from build123d import *

# Parameters (mm, degrees)
F0_R        = 1.1
F1_DEPTH    = 4.75
F2_R        = 5
F3_DEPTH    = 5
F5_T1_DEPTH = 16.1499020619
F5_T3_DEPTH = 14.3297238483
F5_T5_DEPTH = 10.7226436636
F7_DEPTH    = 0.8
F8_R        = 0.75
F9_R        = 9.625
F10_DEPTH   = 3
F12_R       = 4.5172071506
F12_R_2     = 2.2672071506
F13_DEPTH   = 3.7


# Not quite as in the source:
# - a fillet or chamfer that OpenCascade refuses, or shapes differently, is made with other operations: its cross-section is extruded or revolved along the edge and cut away or added


with BuildPart() as f1:
    # F0 (on Top) → F1 (new body)
    with BuildSketch(Plane.XY):
        with BuildLine():
            Line((-8.3357166343, -1.6650899635), (-12.2050748298, -2.6992866465))
            ThreePointArc((-12.2050748298, -2.6992866465), (-9.3300068577, -8.3187121621), (-4.0757746589, -11.8168549509))
            ThreePointArc((-4.0757746589, -11.8168549509), (-3.593311946, -12.8676823003), (-2.8459674038, -13.75))
            Line((-2.8459674038, -13.75), (2.8459674038, -13.75))
            ThreePointArc((2.8459674038, -13.75), (3.593311946, -12.8676823003), (4.0757746589, -11.8168549509))
            ThreePointArc((4.0757746589, -11.8168549509), (9.3300068577, -8.3187121621), (12.2050748298, -2.6992866465))
            Line((12.2050748298, -2.6992866465), (8.3357166343, -1.6650899635))
            ThreePointArc((8.3357166343, -1.6650899635), (8.1313688943, -2.4774051544), (7.8480653995, -3.2656646917))
            ThreePointArc((7.8480653995, -3.2656646917), (8.5179809488, -4.8326547168), (6.82922604, -5.061459087))
            Line((6.82922604, -5.061459087), (5.0334316447, -3.2656646917))
            ThreePointArc((5.0334316447, -3.2656646917), (0, 6), (-5.0334316447, -3.2656646917))
            Line((-5.0334316447, -3.2656646917), (-6.82922604, -5.061459087))
            ThreePointArc((-6.82922604, -5.061459087), (-8.5179809488, -4.8326547168), (-7.8480653995, -3.2656646917))
            ThreePointArc((-7.8480653995, -3.2656646917), (-8.1313688943, -2.4774051544), (-8.3357166343, -1.6650899635))
        make_face()
        with Locations((0, -10.9)):
            Circle(F0_R, mode=Mode.SUBTRACT)
        with BuildLine():
            Line((-5.061459087, -6.82922604), (-3.2656646917, -5.0334316447))
            ThreePointArc((-3.2656646917, -5.0334316447), (0, -6), (3.2656646917, -5.0334316447))
            Line((3.2656646917, -5.0334316447), (5.061459087, -6.82922604))
            ThreePointArc((5.061459087, -6.82922604), (4.8326547168, -8.5179809488), (3.2656646917, -7.8480653995))
            ThreePointArc((3.2656646917, -7.8480653995), (0, -8.5003938964), (-3.2656646917, -7.8480653995))
            ThreePointArc((-3.2656646917, -7.8480653995), (-4.8326547168, -8.5179809488), (-5.061459087, -6.82922604))
        make_face(mode=Mode.SUBTRACT)
    extrude(amount=F1_DEPTH)

    # F2 (on face) → F3 (join)
    with BuildSketch(Plane.XY.offset(4.75)):
        Circle(F2_R)
    extrude(amount=F3_DEPTH)

    # F5: fillet of radius 2 on 6 edges, made by hand

    # F5_s2 → F5_t1 (cut)
    with BuildSketch(Plane.XY.offset(-5.6999510309)):
        with BuildLine():
            ThreePointArc((10.1863028618, -2.1597120795), (11.4666976063, -3.2135797735), (11.5117544763, -4.871294374))
            ThreePointArc((11.5117544763, -4.871294374), (11.9080394052, -3.801131085), (12.2050748298, -2.6992866465))
            Line((12.2050748298, -2.6992866465), (10.1863028618, -2.1597120795))
        make_face()
        with BuildLine():
            ThreePointArc((-10.1863028618, -2.1597120795), (-11.4666976063, -3.2135797735), (-11.5117544763, -4.871294374))
            ThreePointArc((-11.5117544763, -4.871294374), (-11.9080394052, -3.801131085), (-12.2050748298, -2.6992866465))
            Line((-12.2050748298, -2.6992866465), (-10.1863028618, -2.1597120795))
        make_face()
    extrude(amount=F5_T1_DEPTH, mode=Mode.SUBTRACT)

    # F5_s4 → F5_t3 (cut)
    with BuildSketch(Plane.XY.offset(-4.7898619242)):
        with BuildLine():
            ThreePointArc((10.1866871135, -2.1598147817), (8.7919457915, -2.2951684372), (7.8283732011, -3.3125925525))
            ThreePointArc((7.8283732011, -3.3125925525), (8.1239163121, -2.5017354271), (8.3357166343, -1.6650899635))
            Line((8.3357166343, -1.6650899635), (10.1866871135, -2.1598147817))
        make_face()
        with BuildLine():
            ThreePointArc((-7.8283732011, -3.3125925525), (-8.7919457915, -2.2951684372), (-10.1866871135, -2.1598147817))
            Line((-10.1866871135, -2.1598147817), (-8.3357166343, -1.6650899635))
            ThreePointArc((-8.3357166343, -1.6650899635), (-8.1239163121, -2.5017354271), (-7.8283732011, -3.3125925525))
        make_face()
    extrude(amount=F5_T3_DEPTH, mode=Mode.SUBTRACT)

    # F5_s6 → F5_t5 (cut)
    with BuildSketch(Plane.XY.offset(-2.9863218318)):
        with BuildLine():
            ThreePointArc((3.7221531416, -8.4854887571), (2.954728203, -8.190033245), (2.1332864048, -8.2283525392))
            ThreePointArc((2.1332864048, -8.2283525392), (2.7061638555, -8.0581246938), (3.2656646917, -7.8480653995))
            ThreePointArc((3.2656646917, -7.8480653995), (3.4334814116, -8.2100520192), (3.7221531416, -8.4854887571))
        make_face()
        with BuildLine():
            ThreePointArc((-2.1332864048, -8.2283525392), (-2.954728203, -8.190033245), (-3.7221531416, -8.4854887571))
            ThreePointArc((-3.7221531416, -8.4854887571), (-3.4334814116, -8.2100520192), (-3.2656646917, -7.8480653995))
            ThreePointArc((-3.2656646917, -7.8480653995), (-2.7061638555, -8.0581246938), (-2.1332864048, -8.2283525392))
        make_face()
    extrude(amount=F5_T5_DEPTH, mode=Mode.SUBTRACT)

    # F6 (on face) → F7 (cut)
    with BuildSketch(Plane.XY.offset(4.75)):
        Polygon((4.377220794, -8.6198614811), (8.6198614811, -4.377220794), (7.0098197866, -2.8055128878), (2.7863459937, -7.0289866808), align=None)
        Polygon((-4.377220794, -8.6198614811), (-2.7863459937, -7.0289866808), (-7.0098197866, -2.8055128878), (-8.6198614811, -4.377220794), align=None)
    extrude(amount=-F7_DEPTH, mode=Mode.SUBTRACT)

    # F8
    f8_edges = [f1.edges().sort_by_distance(p)[0] for p in [
        (4.907666, -4.907666, 3.95),
        (-4.907666, -4.907666, 3.95),
        (-5, 0, 4.75),
        (-5, 0, 9.75),
    ]]
    fillet(f8_edges, radius=F8_R)

    # F9 (on Top) → F10 (cut)
    with BuildSketch(Plane.XY):
        Circle(F9_R)
    extrude(amount=F10_DEPTH, mode=Mode.SUBTRACT)

    # F12 (on face) → F13 (cut)
    with BuildSketch(Plane(origin=(0, 0, 3), x_dir=(1, 0, 0), z_dir=(0, 0, -1))):
        Circle(F12_R)
        Circle(F12_R_2, mode=Mode.SUBTRACT)
    extrude(amount=-F13_DEPTH, mode=Mode.SUBTRACT)


solid = f1.part
Build history of the part. All positions in model axes, mm. A direction names the side the tool comes from. Coordinates: 2 decimals unless noted, no trailing zeros. Order: outer loops, then holes, each group sorted by start corner. A loop starts at its lowest first (then second) coordinate and runs counter-clockwise, first axis right, second up. Notation, with made-up numbers: (76.5, 66) - (91.5, 66) arc R28 cw to (91.5, 93) - close; hole circle Ø2 at (74.5, 77.25). An arc over 180 degrees is marked (long way). Write item = value, one per line. Start each with the question number.
1) Saw through at D-D on y = 0. Write the cut outline in (x, z), then the cut area to 4 significant figures.
2) Saw through at C-C on y = -10.9. Write the cut outline in (x, z), then the cut area to 3 significant figures.
3) Two-plate mould, pull along Y, no slides. Class faces 5 (the face through (0, -9, 4.75)), 6 (the face through (0, -13.75, 2)), 7 (the face through (2.966, -8.192, 3.863)): pulls with the +Y half, pulls with the -Y half, needs draft (parallel to the pull), parting line crosses it, or undercut.
4) Wall check: line 1 along X through (y, z) = (-0.5, 3.75); line 2 along Y through (x, z) = (0, 5); line 3 along Z through (x, y) = (1.75, 0.5). Give the ranges that are in metal, low to high. Write a range as from..to.
5) 3-axis set-ups, long thin cutter, end or side, ignore diameter. For faces 1 (the face through (3.95, -5.72, 3.67)), 2 (the face through (-6.514, -6.483, 4.356)), 3 (the face through (8.6, -2.9, 3)), 4 (the face through (2, 2, 6.7)): which of +Z, -Z, +X, -X, +Y, -Y reach the whole face in a straight line?
6) Saw through at A-A on x = 0. Count the separate pieces of the cut face and the enclosed holes in it, then the cut area to 3 significant figures.
7) Flat gauge pins, fed straight in: pin 1 Ø2.5 at (x, y) = (1.5, 0) entering from -Z; pin 2 Ø1 at (x, z) = (5, 4) entering from -Y; pin 3 Ø3 at (y, z) = (-6, 5) entering from -X; pin 4 Ø1.7 at (x, y) = (-8.5, -3.5) entering from -Z. Where does each tip first touch, or does it go through?
From the geometry:
q1.outline = (-6, 3) - (-4.52, 3) - (-4.52, 6.7) - (-2.27, 6.7) - (-2.27, 3) - (2.27, 3) - (2.27, 6.7) - (4.52, 6.7) - (4.52, 3) - (6, 3) - (6, 4.75) - (5.75, 4.75) arc R0.75 cw to (5, 5.5) - (5, 9) arc R0.75 ccw to (4.25, 9.75) - (-4.25, 9.75) arc R0.75 ccw to (-5, 9) - (-5, 5.5) arc R0.75 cw to (-5.75, 4.75) - (-6, 4.75) - close
q1.area = 54.35 mm^2
q2.outline = (-6.12, 0) - (-1.1, 0) - (-1.1, 4.75) - (-6.12, 4.75) - close; (1.1, 0) - (6.12, 0) - (6.12, 4.75) - (1.1, 4.75) - close
q2.area = 47.7 mm^2
q3.face_5 = needs draft
q3.face_6 = pulls with the -Y half
q3.face_7 = undercut
q4.line_1 = -5.98..-4.49, -2.21..2.21, 4.49..5.98
q4.line_2 = -5.19..-4.52, -2.27..2.27, 4.52..5.19
q4.line_3 = 3..9.75
q5.face_1 = +Z, -Z
q5.face_2 = +Z
q5.face_3 = -Z, +Y
q5.face_4 = -Z
q6.separate_pieces = 3
q6.enclosed_holes = 0
q6.area = 65.5 mm^2
q7.pin_1 = 3
q7.pin_2 = -11.66
q7.pin_3 = -11.62
q7.pin_4 = 0
